Build history of the part. All positions in model axes, mm. A direction names the side the tool comes from. Round coordinates to 2 decimals unless told otherwise and drop trailing zeros. Loops run counter-clockwise (first coordinate to the right, second up) from the corner with the lowest first, then second, coordinate; pieces in that order, holes last. Notation, with made-up numbers: (11.25, -24.5) - (18.25, -24.5) arc R22 ccw to (18.25, -1.5) - close; hole circle Ø2 at (41, 33.5). An arc over 180 degrees is marked (long way). Answer as CSV lines item,"result". Start each with the question number.
```python
from build123d import *

# Parameters (mm, degrees)
BOX003_W                = 300
BOX003_H                = 300
BOX003_DEPTH            = 100
BOX002_W                = 300
BOX002_H                = 300
BOX002_DEPTH            = 100
CYLINDER006_R           = 11
CYLINDER006_DEPTH       = 68
CYLINDER006_PITCH_ANGLE = 90
CYLINDER007_R           = 4
CYLINDER007_DEPTH       = 72
CYLINDER007_ROLL_ANGLE  = 90
SKETCH003_R             = 16.230199
PAD002_DEPTH            = 60
SKETCH002_W             = 75.068111
SKETCH002_H             = 10.178723
PAD003_DEPTH            = 60
FILLET_R                = 7
FILLET001_R             = 7
FILLET002_R             = 7


with BuildPart() as cube003:
    # Box003 → Box003 (new body)
    with BuildSketch(Plane(origin=(-150, -150, 23), x_dir=(1, 0, 0), z_dir=(0, 0, 1))):
        with Locations((150, 150)):
            Rectangle(BOX003_W, BOX003_H)
    extrude(amount=BOX003_DEPTH)


with BuildPart() as fusion002:
    # Box002 → Box002 (new body)
    with BuildSketch(Plane(origin=(-150, -150, -102), x_dir=(1, 0, 0), z_dir=(0, 0, 1))):
        with Locations((150, 150)):
            Rectangle(BOX002_W, BOX002_H)
    extrude(amount=BOX002_DEPTH)

    # Fusion002: union Cube003
    add(cube003.part)


with BuildPart() as cylindre005:
    # Cylinder006 → Cylinder006 (new body)
    with BuildSketch(Plane.XY):
        Circle(CYLINDER006_R)
    extrude(amount=CYLINDER006_DEPTH)


with BuildPart() as cylindre005_1:
    # Cylinder006 pitch: moved
    add(cylindre005.part.rotate(Axis((0, 0, 0), (0, 1, 0)), CYLINDER006_PITCH_ANGLE))


with BuildPart() as cylindre005_2:
    # Cylinder006 placement: moved
    add(cylindre005_1.part.moved(Location((-32, 0, 10.5))))


with BuildPart() as obj1:
    # Sphere001 → Sphere001 (revolve)
    with BuildSketch(Plane(origin=(0, 0, 10.5), x_dir=(1, 0, 0), z_dir=(0, -1, 0))):
        with BuildLine():
            ThreePointArc((0, -21.2), (21.2, 0), (0, 21.2))
            Line((0, 21.2), (0, -21.2))
        make_face()
    revolve(axis=Axis((0, 0, 10.5), (0, 0, 1)))


with BuildPart() as cut008:
    # Sphere002 → Sphere002 (revolve)
    with BuildSketch(Plane(origin=(0, 0, 10.5), x_dir=(1, 0, 0), z_dir=(0, -1, 0))):
        with BuildLine():
            ThreePointArc((0, -27.1), (27.1, 0), (0, 27.1))
            Line((0, 27.1), (0, -27.1))
        make_face()
    revolve(axis=Axis((0, 0, 10.5), (0, 0, 1)))

    # Cut006: cut obj1
    add(obj1.part, mode=Mode.SUBTRACT)

    # Cut007: cut Cylindre005
    add(cylindre005_2.part, mode=Mode.SUBTRACT)

    # Cut008: cut Fusion002
    add(fusion002.part, mode=Mode.SUBTRACT)


with BuildPart() as obj2:
    # Sphere003 → Sphere003 (revolve)
    with BuildSketch(Plane(origin=(0, 0, 10.5), x_dir=(1, 0, 0), z_dir=(0, -1, 0))):
        with BuildLine():
            ThreePointArc((0, -21.4), (21.4, 0), (0, 21.4))
            Line((0, 21.4), (0, -21.4))
        make_face()
    revolve(axis=Axis((0, 0, 10.5), (0, 0, 1)))


with BuildPart() as obj3:
    # Cylinder007 → Cylinder007 (new body)
    with BuildSketch(Plane.XY):
        Circle(CYLINDER007_R)
    extrude(amount=CYLINDER007_DEPTH)


with BuildPart() as obj3_1:
    # Cylinder007 roll: moved
    add(obj3.part.rotate(Axis((0, 0, 0), (1, 0, 0)), CYLINDER007_ROLL_ANGLE))


with BuildPart() as obj3_2:
    # Cylinder007 placement: moved
    add(obj3_1.part.moved(Location((0, 36, 10.5))))

    # Cut009: cut obj2
    add(obj2.part, mode=Mode.SUBTRACT)

    # Fusion003: union Cut008
    add(cut008.part)


with BuildPart() as pad002:
    # Sketch003 → Pad002 (new body)
    with BuildSketch(Plane.YZ.offset(-25)):
        with Locations((0.508931, 9.669792)):
            Circle(SKETCH003_R)
    extrude(amount=PAD002_DEPTH)


with BuildPart() as medium2:
    # Sketch002 → Pad003 (new body)
    with BuildSketch(Plane.YZ.offset(-25)):
        with Locations((0.127233, 9.924257)):
            Rectangle(SKETCH002_W, SKETCH002_H)
    extrude(amount=PAD003_DEPTH)

    # Fusion007: union Pad002
    add(pad002.part)

    # Common002: intersect obj3
    add(obj3_2.part, mode=Mode.INTERSECT)

    # Fillet
    fillet_edges = [medium2.edges().sort_by_distance(p)[0] for p in [
        (18.017556, 9.767706, 23),
        (-18.017556, 9.767706, 23),
    ]]
    fillet(fillet_edges, radius=FILLET_R)

    # Fillet001
    fillet001_edges = [medium2.edges().sort_by_distance(p)[0] for p in [
        (-18.557399, -8.749844, 23),
        (18.557399, -8.749844, 23),
    ]]
    fillet(fillet001_edges, radius=FILLET001_R)

    # Fillet002
    fillet002_edges = [medium2.edges().sort_by_distance(p)[0] for p in [
        (-17.404195, -10.770932, -2),
        (17.404195, -10.770932, -2),
        (16.687516, 11.788794, -2),
        (-16.687516, 11.788794, -2),
    ]]
    fillet(fillet002_edges, radius=FILLET002_R)


solid = medium2.part
```
Q1. Band-saw the part on C-C, the plane y = -3. List the corners of the cut face in (x, z).
Q2. Two-plate mould, pull along Z, no slides. Class faces 5 (the flat face through (0, 21, 4.835)), 6 (the flat face through (-20, 1, 23)), 7 (the cylindrical face through (-21.49, -10.74, 12.88)): released by +Z, released by -Z, zero draft, split by the parting line, or undercut.
Q3. Band-saw the part on D-D, the plane z = 3.25. List the corners of the cut face in (x, y), then the cut area to 3 significant figures.
Q4. Tool access for faces 1 (the cylindrical face through (-0.521, 31.466, 14.466)), 2 (the flat face through (0, 21, 15.014)), 3 (the flat face through (0, -21, 4.835)), 4 (the cylindrical face through (-0.867, -31.337, 6.595)): list every direction of +Z, -Z, +X, -X, +Y, -Y with a clear straight run to the whole face (end or side of a thin tool).
Q5. Band-saw the part on A-A, the plane z = 10.5. List the corners of the cut face in (x, y).
Q6. Wall check: probe 1 along Z at (x, y) = (19, 0); probe 2 along X at (y, z) = (16.5, 5); probe 3 along Y at (x, z) = (-19.25, 10.5). Give the ranges that are in metal, low to high. Write a range as [from, to].
Q7. Band-saw the part on B-B, the plane x = 0. List the corners of the cut face in (y, z).
Q8. Pin check, flat tips, straight feed: pin 1 Ø4 at (x, y) = (12.5, -12) entering from +Z; pin 2 Ø3.5 at (x, y) = (-8.5, 21.5) entering from +Z; pin 3 Ø3 at (x, y) = (-10, 21) entering from -Z. Stop position of each tip, or through.
Reported:
1,outline,"(-24.77, -0.08) arc R26.93 ccw to (-23.86, -2) - (-16.86, -2) arc R20.99 cw to (-18.12, -0.08) - close; (-24.77, 21.08) - (-18.12, 21.08) arc R20.99 cw to (-16.86, 23) - (-23.86, 23) arc R26.93 ccw to start; (16.86, -2) - (23.86, -2) arc R26.93 ccw to (24.77, -0.08) - (18.12, -0.08) arc R20.99 cw to start; (16.86, 23) arc R20.99 cw to (18.12, 21.08) - (24.77, 21.08) arc R26.93 ccw to (23.86, 23) - close"
2,face 5,"released by -Z"
2,face 6,"released by +Z"
2,face 7,"undercut"
3,outline,"(-24.77, -8.27) arc R26.11 ccw to (-21.78, -14.4) - (-13.77, -14.4) arc R19.92 cw to (-18.12, -8.27) - close; (-24.77, 8.27) - (-18.12, 8.27) arc R19.92 cw to (-12.62, 15.42) - (-21.08, 15.42) arc R26.11 ccw to start; (12.62, 15.42) arc R19.92 cw to (18.12, 8.27) - (24.77, 8.27) arc R26.11 ccw to (21.08, 15.42) - close; (13.77, -14.4) - (21.78, -14.4) arc R26.11 ccw to (24.77, -8.27) - (18.12, -8.27) arc R19.92 cw to start"
3,area,"193 mm2"
4,face 1,"+Y"
4,face 2,"+Z, +X, -X, +Y"
4,face 3,"-Z, +X, -X, -Y"
4,face 4,"-Y"
5,outline,"(-24.77, -11) arc R27.1 ccw to (-4, -26.8) - (-4, -36) - (4, -36) - (4, -26.8) arc R27.1 ccw to (24.77, -11) - (18.12, -11) arc R21.2 cw to (-18.12, -11) - close; (-24.77, 11) - (-18.12, 11) arc R21.2 cw to (18.12, 11) - (24.77, 11) arc R27.1 ccw to (4, 26.8) - (4, 36) - (-4, 36) - (-4, 26.8) arc R27.1 ccw to start"
6,probe 1,"z = [-2, -0.5], [21.5, 23]"
6,probe 2,"x = [-20.78, -12.12], [12.12, 20.78]"
6,probe 3,"y = [-19.07, -11], [11, 19.07]"
7,outline,"(-36, 6.5) - (-26.8, 6.5) arc R27.1 ccw to (-26.5, 4.83) - (-20.43, 4.83) arc R21.2 cw to (-20.71, 15.01) - (-26.72, 15.01) arc R27.1 ccw to (-26.8, 14.5) - (-36, 14.5) - close; (20.43, 4.83) - (26.5, 4.83) arc R27.1 ccw to (26.8, 6.5) - (36, 6.5) - (36, 14.5) - (26.8, 14.5) arc R27.1 ccw to (26.72, 15.01) - (20.71, 15.01) arc R21.2 cw to start"
8,pin 1,"stops at z = 1.79"
8,pin 2,"stops at z = 15.01"
8,pin 3,"stops at z = 4.83"
